Check sheet for the modelled part. Datum: model origin and axes. Units: mm. A direction names the side the tool comes from. Give positions to 0.01 mm unless a question says otherwise; leave off trailing zeros. Write each loop counter-clockwise with the first axis right and the second up, starting at its lowest first coordinate (ties: lowest second). Pieces come first, ordered by that corner, then holes. Notation, with made-up numbers: (0.25, 74) - (37.25, 74) arc R17 cw to (37.25, 104) - close; hole circle Ø3 at (-21.75, 28.5). An arc over 180 degrees is marked (long way). Return JSON: item names as keys, results as strings. Group by question number.
```python
from build123d import *
from OCP.BRepFilletAPI import BRepFilletAPI_MakeChamfer

# Parameters (mm, degrees)
DODANIE_WYCI_GNI_CIE1_DEPTH = 6.5
DODANIE_WYCI_GNI_CIE2_DEPTH = 3
SFAZOWANIE1_SIZE            = 1
SFAZOWANIE1_SIZE2           = 2.747477419


with BuildPart() as part:
    # Szkic2 → Dodanie-wyciągnięcie1 (new body)
    with BuildSketch(Plane.XY):
        with BuildLine():
            Line((-39.650742014, 108.939518347), (-32.120772186, 88.251096277))
            ThreePointArc((-32.120772186, 88.251096277), (-30.12924195, 86.030742386), (-27.155108014, 85.805594857))
            ThreePointArc((-27.155108014, 85.805594857), (-13.738567299, 88.945217795), (0, 90))
            Line((0, 90), (0, 120))
            ThreePointArc((0, 120), (-18.796846712, 118.518684408), (-37.129625721, 114.111309228))
            ThreePointArc((-37.129625721, 114.111309228), (-39.48751323, 112.060333895), (-39.650742014, 108.939518347))
        make_face()
    dodanie_wyci_gni_cie1 = extrude(amount=DODANIE_WYCI_GNI_CIE1_DEPTH)

    # Szkic3 → Dodanie-wyciągnięcie2 (add)
    with BuildSketch(Plane.XY.offset(6.5)):
        with BuildLine():
            Line((-46, 91), (-35.249646863, 91))
            Line((-35.249646863, 91), (-34.000157428, 87.567055991))
            ThreePointArc((-34.000157428, 87.567055991), (-31.012862074, 84.236525153), (-26.551661169, 83.89880386))
            ThreePointArc((-26.551661169, 83.89880386), (-13.433265804, 86.968657399), (0, 88))
            Line((0, 88), (0, 90))
            ThreePointArc((0, 90), (-13.738567299, 88.945217795), (-27.155108014, 85.805594857))
            ThreePointArc((-27.155108014, 85.805594857), (-30.12924195, 86.030742386), (-32.120772186, 88.251096277))
            Line((-32.120772186, 88.251096277), (-39.650742014, 108.939518347))
            ThreePointArc((-39.650742014, 108.939518347), (-39.48751323, 112.060333895), (-37.129625721, 114.111309228))
            ThreePointArc((-37.129625721, 114.111309228), (-18.796846712, 118.518684408), (0, 120))
            Line((0, 120), (0, 122))
            ThreePointArc((0, 122), (-19.11012749, 120.493995814), (-37.748452817, 116.013164382))
            ThreePointArc((-37.748452817, 116.013164382), (-41.285284079, 112.936701382), (-41.530127255, 108.255478061))
            Line((-41.530127255, 108.255478061), (-39.617289674, 103))
            Line((-39.617289674, 103), (-46, 103))
            Line((-46, 103), (-46, 106.5))
            ThreePointArc((-46, 106.5), (-46.146446609, 106.853553391), (-46.5, 107))
            Line((-46.5, 107), (-48.5, 107))
            ThreePointArc((-48.5, 107), (-48.853553391, 106.853553391), (-49, 106.5))
            Line((-49, 106.5), (-49, 103))
            Line((-49, 103), (-49, 85.5))
            ThreePointArc((-49, 85.5), (-48.853553391, 85.146446609), (-48.5, 85))
            Line((-48.5, 85), (-46.5, 85))
            ThreePointArc((-46.5, 85), (-46.146446609, 85.146446609), (-46, 85.5))
            Line((-46, 85.5), (-46, 91))
        make_face()
        with BuildLine():
            ThreePointArc((-27.155108014, 85.805594857), (-13.738567299, 88.945217795), (0, 90))
            Line((0, 90), (0, 120))
            ThreePointArc((0, 120), (-18.796846712, 118.518684408), (-37.129625721, 114.111309228))
            ThreePointArc((-37.129625721, 114.111309228), (-39.48751323, 112.060333895), (-39.650742014, 108.939518347))
            Line((-39.650742014, 108.939518347), (-32.120772186, 88.251096277))
            ThreePointArc((-32.120772186, 88.251096277), (-30.12924195, 86.030742386), (-27.155108014, 85.805594857))
        make_face()
    dodanie_wyci_gni_cie2 = extrude(amount=DODANIE_WYCI_GNI_CIE2_DEPTH)

    # Lustro1: Dodanie-wyciągnięcie1, Dodanie-wyciągnięcie2 across plane
    add(dodanie_wyci_gni_cie1.mirror(Plane(origin=(0, 0, 0), x_dir=(0, 0, 1), z_dir=(1, 0, 0))))
    add(dodanie_wyci_gni_cie2.mirror(Plane(origin=(0, 0, 0), x_dir=(0, 0, 1), z_dir=(1, 0, 0))))

    # Sfazowanie1: one chamfer whose edges measure the first distance from different faces: ONE call of the kernel's chamfer builder (chamfer() names one face for all edges)
    sfazowanie1_edges_1 = [part.edges().sort_by_distance(p)[0] for p in [
        (-39.48751323, 112.060333895, 0),
    ]]
    sfazowanie1_side_1 = [part.faces().sort_by_distance(p)[0] for p in [
        (-39.48751323, 112.060333895, 3.25),
    ]]
    sfazowanie1_edges_2 = [part.edges().sort_by_distance(p)[0] for p in [
        (0, 120, 0),
    ]]
    sfazowanie1_side_2 = [part.faces().sort_by_distance(p)[0] for p in [
        (0, 120, 3.25),
    ]]
    sfazowanie1_edges_3 = [part.edges().sort_by_distance(p)[0] for p in [
        (30.12924195, 86.030742386, 0),
    ]]
    sfazowanie1_side_3 = [part.faces().sort_by_distance(p)[0] for p in [
        (30.12924195, 86.030742386, 3.25),
    ]]
    sfazowanie1_edges_4 = [part.edges().sort_by_distance(p)[0] for p in [
        (35.8857571, 98.595307312, 0),
    ]]
    sfazowanie1_side_4 = [part.faces().sort_by_distance(p)[0] for p in [
        (35.8857571, 98.595307312, 3.25),
    ]]
    sfazowanie1_edges_5 = [part.edges().sort_by_distance(p)[0] for p in [
        (39.48751323, 112.060333895, 0),
    ]]
    sfazowanie1_side_5 = [part.faces().sort_by_distance(p)[0] for p in [
        (39.48751323, 112.060333895, 3.25),
    ]]
    sfazowanie1_edges_6 = [part.edges().sort_by_distance(p)[0] for p in [
        (0, 90, 0),
    ]]
    sfazowanie1_side_6 = [part.faces().sort_by_distance(p)[0] for p in [
        (0, 90, 3.25),
    ]]
    sfazowanie1_edges_7 = [part.edges().sort_by_distance(p)[0] for p in [
        (-30.12924195, 86.030742386, 0),
    ]]
    sfazowanie1_side_7 = [part.faces().sort_by_distance(p)[0] for p in [
        (-30.12924195, 86.030742386, 3.25),
    ]]
    sfazowanie1_edges_8 = [part.edges().sort_by_distance(p)[0] for p in [
        (-35.8857571, 98.595307312, 0),
    ]]
    sfazowanie1_side_8 = [part.faces().sort_by_distance(p)[0] for p in [
        (-35.8857571, 98.595307312, 3.25),
    ]]
    sfazowanie1 = BRepFilletAPI_MakeChamfer(part.part.solid().wrapped)
    for e in sfazowanie1_edges_1:
        sfazowanie1.Add(SFAZOWANIE1_SIZE, SFAZOWANIE1_SIZE2, e.wrapped, sfazowanie1_side_1[0].wrapped)  # the first distance lies on this face
    for e in sfazowanie1_edges_2:
        sfazowanie1.Add(SFAZOWANIE1_SIZE, SFAZOWANIE1_SIZE2, e.wrapped, sfazowanie1_side_2[0].wrapped)  # the first distance lies on this face
    for e in sfazowanie1_edges_3:
        sfazowanie1.Add(SFAZOWANIE1_SIZE, SFAZOWANIE1_SIZE2, e.wrapped, sfazowanie1_side_3[0].wrapped)  # the first distance lies on this face
    for e in sfazowanie1_edges_4:
        sfazowanie1.Add(SFAZOWANIE1_SIZE, SFAZOWANIE1_SIZE2, e.wrapped, sfazowanie1_side_4[0].wrapped)  # the first distance lies on this face
    for e in sfazowanie1_edges_5:
        sfazowanie1.Add(SFAZOWANIE1_SIZE, SFAZOWANIE1_SIZE2, e.wrapped, sfazowanie1_side_5[0].wrapped)  # the first distance lies on this face
    for e in sfazowanie1_edges_6:
        sfazowanie1.Add(SFAZOWANIE1_SIZE, SFAZOWANIE1_SIZE2, e.wrapped, sfazowanie1_side_6[0].wrapped)  # the first distance lies on this face
    for e in sfazowanie1_edges_7:
        sfazowanie1.Add(SFAZOWANIE1_SIZE, SFAZOWANIE1_SIZE2, e.wrapped, sfazowanie1_side_7[0].wrapped)  # the first distance lies on this face
    for e in sfazowanie1_edges_8:
        sfazowanie1.Add(SFAZOWANIE1_SIZE, SFAZOWANIE1_SIZE2, e.wrapped, sfazowanie1_side_8[0].wrapped)  # the first distance lies on this face
    add(Compound.cast(sfazowanie1.Shape()), mode=Mode.REPLACE)


solid = part.part
```
Item 1: Access from +Z, -Z, +X, -X, +Y, -Y to the whole of each face (thin tool, end or side, straight path). Record for faces 1 (the face through (-30.17, 86.05, 3.71)), 2 (the face through (-39.47, 112.1, 3.71)), 3 (the face through (-35.94, 98.74, 3.71)).
Item 2: Mould release check, pull along Y, two halves, no side actions. Record for faces 4 (the face through (30.17, 86.05, 3.71)), 5 (the face through (41.255, 112.997, 7.979)), 6 (the face through (-49, 96, 8)): +Y half, -Y half, draft (parallel to the pull), parting line (faces both ways), or undercut.
Item 3: Depth check by flat-ended pin: pin 1 (1.6 mm diameter, centred on x = -47.5, z = 8, fed in from +Y); pin 2 (2.5 mm diameter, centred on x = 42.5, z = 8, fed in from +Y); pin 3 (3 mm diameter, centred on y = 95, z = 2.5, fed in from +X). Enter the tip coordinate at first touch or a pass-through.
Item 4: Section check B-B on y = 105.5. Record the cut outline in (x, z).
Item 5: Material ranges on line 1 along X through (y, z) = (90, 8); line 2 along X through (y, z) = (110, 6.25); line 3 along Y through (x, z) = (-1, 3.5), recorded low to high. Write a range as from..to.
Reply:
{
 "1": {"face 1": "-Z, -Y", "face 2": "-Z, -X", "face 3": "-Z, -X, -Y"},
 "2": {"face 4": "-Y half", "face 5": "undercut", "face 6": "draft"},
 "3": {"pin 1": "y = 107", "pin 2": "y = 113.01", "pin 3": "x = 35.12"},
 "4": {"outline": "(-49, 6.5) - (-46, 6.5) - (-46, 9.5) - (-49, 9.5) - close; (-40.53, 6.5) - (-38.4, 6.5) - (-38.4, 1) - (-35.48, 0) - (35.48, 0) - (38.4, 1) - (38.4, 6.5) - (40.53, 6.5) - (40.53, 9.5) - (-40.53, 9.5) - close; (46, 6.5) - (49, 6.5) - (49, 9.5) - (46, 9.5) - close"},
 "5": {"line 1": "-49..-46, -34.89..34.89, 46..49", "line 2": "-39.88..39.88", "line 3": "89.99..120"}
}
